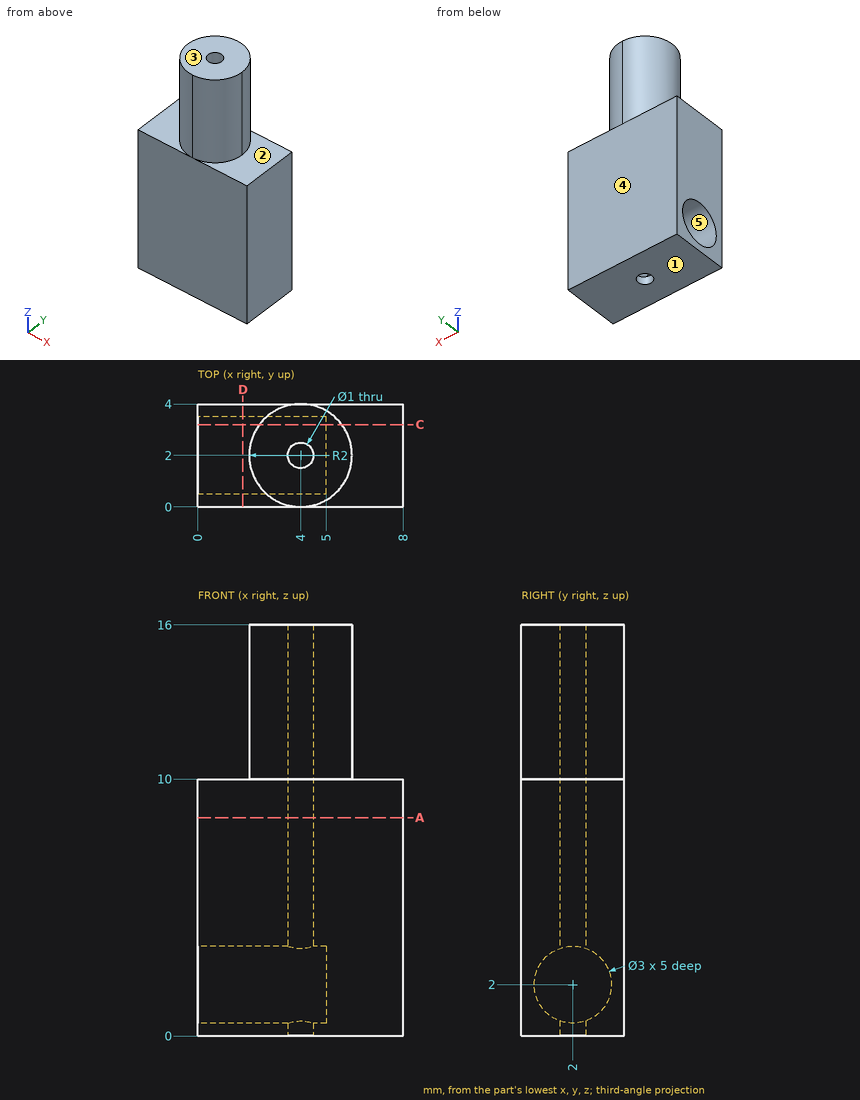
Check sheet for the drawn part. Datum: minimum x, y, z corner. Units: mm. A direction names the side the tool comes from. Give positions to 0.01 mm unless a question says otherwise; leave off trailing zeros. Loops run counter-clockwise (first coordinate to the right, second up) from the corner with the lowest first, then second, coordinate; pieces in that order, holes last. Notation, with made-up numbers: M 68.5,-5.5 L 115.5,-5.5 A17 cw 115.5,5.5 Z; hole C 89.5,48.25 d3. An arc over 180 degrees is marked long. Answer as CSV lines item,"result".
Item 1: Scan lines: L1, parallel to Y at x = 4, z = 9.5; L2, parallel to Z at x = 6.5, y = 0.85; L3, parallel to X at y = 2.2, z = 12.5. Record each from-to range of solid material in increasing order.
Reply:
L1,"0 to 1.5, 2.5 to 4"
L2,"0 to 10"
L3,"2.01 to 3.54, 4.46 to 5.99"
Item 2: Draft check along Y on the marked faces 3, 4 and 5. Enter one of: pulls with the +Y half, pulls with the -Y half, needs draft (parallel to the pull), parting line crosses it, or undercut.
Reply:
face 3,"needs draft"
face 4,"pulls with the +Y half"
face 5,"undercut"
Item 3: Sectioned sample at A-A, the plane z = 8.5. Enter the section's corners in (x, y), then the cut area to 3 significant figures.
Reply:
outline,"M 0,0 L 8,0 L 8,4 L 0,4 Z; hole C 4,2 d1"
area,"31.2 mm^2"
Item 4: Sectioned sample at C-C, the plane y = 3.2. Enter the section's corners in (x, z).
Reply:
outline,"M 0,0 L 8,0 L 8,10 L 5.6,10 L 5.6,16 L 2.4,16 L 2.4,10 L 0,10 L 0,2.9 L 5,2.9 L 5,1.1 L 0,1.1 Z"
Item 5: Depth check by flat-ended pin: pin 1 Ø2 at (x, y) = (1.5, 1.5) entering from +Z. Enter the tip coordinate at first touch or a pass-through.
Reply:
pin 1,"z = 16"
Item 6: Sectioned sample at D-D, the plane x = 1.75. Enter the section's corners in (y, z), then the cut area to 3 significant figures.
Reply:
outline,"M 0,0 L 4,0 L 4,10 L 0,10 Z; hole C 2,2 d3"
area,"32.9 mm^2"
Item 7: Set-up check for the marked faces 1 and 2: record each of +Z, -Z, +X, -X, +Y, -Y from which the full face is reachable in a straight line by a thin tool's end or side.
Reply:
face 1,"-Z, +X, -X, +Y, -Y"
face 2,"+Z, +X"
